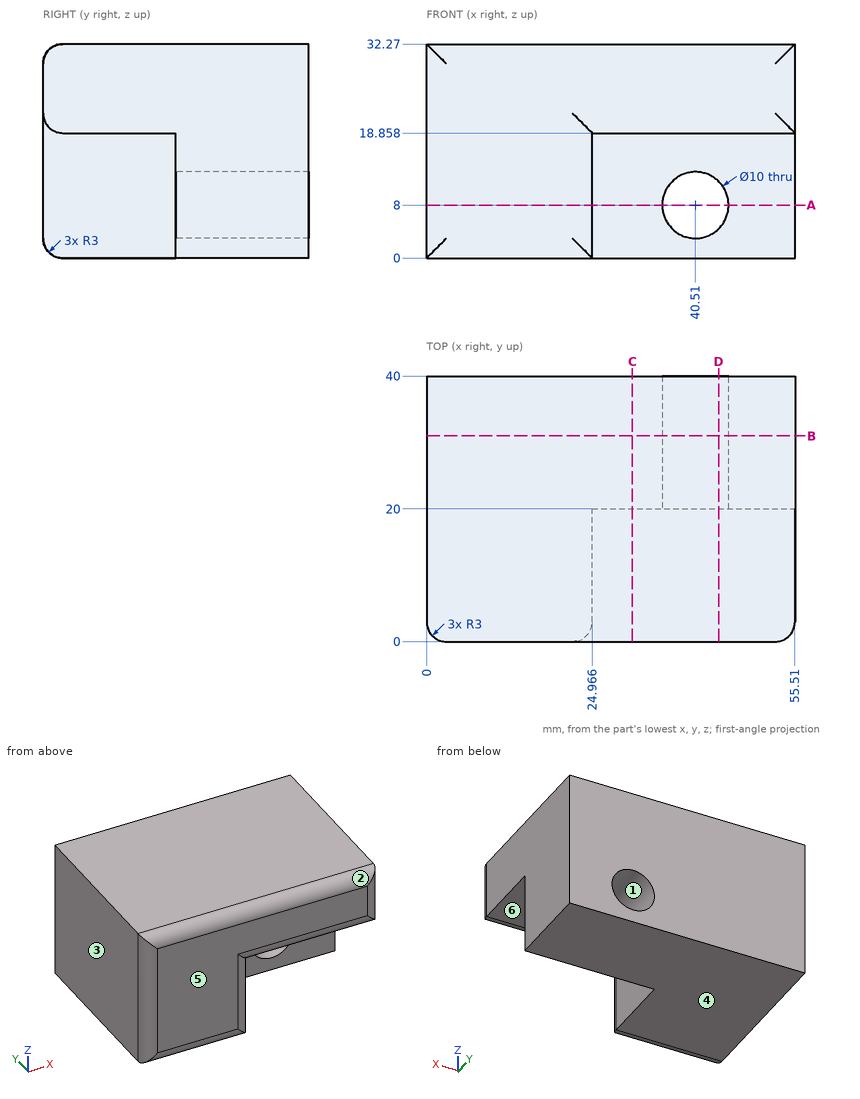
Geometry check sheet. Reference: drawing and pictorial views, mm from the part's lowest x, y, z. A direction names the side the tool comes from. Round coordinates to 2 decimals unless told otherwise and drop trailing zeros. Write each loop counter-clockwise with the first axis right and the second up, starting at its lowest first coordinate (ties: lowest second). Pieces come first, ordered by that corner, then holes. Notation, with made-up numbers: (-22, 2.25) -> (8, 2.25) arc R11 ccw to (8, 23.25) -> close; hole circle Ø4 at (68.25, -18). An arc over 180 degrees is marked (long way). Answer as CSV lines item,"result". Start each with the question number.
1) Material ranges on line 1 (X direction, y = 33.5, z = 8); line 2 (X direction, y = 18, z = 11); line 3 (Y direction, x = 27, z = 9.5), recorded low to high. Write a range as from..to.
2) Section check B-B on y = 31. Enter the section's corners in (x, z), and give its area (3 significant figures).
3) Section check C-C on x = 31. Enter the section's corners in (y, z), and give its area (3 significant figures).
4) Section check D-D on x = 44. Enter the section's corners in (y, z).
5) Section check A-A on z = 8. Enter the section's corners in (x, y).
6) Tool access check on the marked faces 5 and 6. Record the directions out of +Z, -Z, +X, -X, +Y, -Y that give a thin tool (end or side, any length) a straight path to the whole face; none if there is none.
7) Go/stop test with flat-tipped pins: P1, Ø5.5, axis at x = 35, z = 8.5, coming from the -Y side; P2, Ø8.5, axis at y = 14, z = 5, coming from the +X side; P3, Ø8.5, axis at x = 41, y = 9.5, coming from the -Z side. Record where each tip stops, or that it passes through.
8) Release check for a two-part mould opening along Z. For the marked faces 1, 2, 3 and 4 record: pulls with the +Z half, pulls with the -Z half, needs draft (parallel to the pull), parting line crosses it, or undercut.
Found:
1,line 1,"x = 0..35.51, 45.51..55.51"
1,line 2,"x = 0..24.97"
1,line 3,"y = 20..40"
2,outline,"(0, 0) -> (55.51, 0) -> (55.51, 32.27) -> (0, 32.27) -> close; hole circle Ø10 at (40.51, 8)"
2,area,"1,710 mm^2"
3,outline,"(0, 21.86) arc R3 ccw to (3, 18.86) -> (20, 18.86) -> (20, 0) -> (40, 0) -> (40, 32.27) -> (3, 32.27) arc R3 ccw to (0, 29.27) -> close"
3,area,"910 mm^2"
4,outline,"(0, 21.86) arc R3 ccw to (3, 18.86) -> (20, 18.86) -> (20, 11.58) -> (40, 11.58) -> (40, 32.27) -> (3, 32.27) arc R3 ccw to (0, 29.27) -> close; (20, 0) -> (40, 0) -> (40, 4.42) -> (20, 4.42) -> close"
5,outline,"(0, 3) arc R3 ccw to (3, 0) -> (21.97, 0) arc R3 ccw to (24.97, 3) -> (24.97, 20) -> (35.51, 20) -> (35.51, 40) -> (0, 40) -> close; (45.51, 20) -> (55.51, 20) -> (55.51, 40) -> (45.51, 40) -> close"
6,face 5,"+Z, -Z, +X, -X, -Y"
6,face 6,"-Z, +X, -Y"
7,P1,"stops at y = 20"
7,P2,"stops at x = 24.97"
7,P3,"stops at z = 18.86"
8,face 1,"undercut"
8,face 2,"pulls with the +Z half"
8,face 3,"needs draft"
8,face 4,"pulls with the -Z half"
